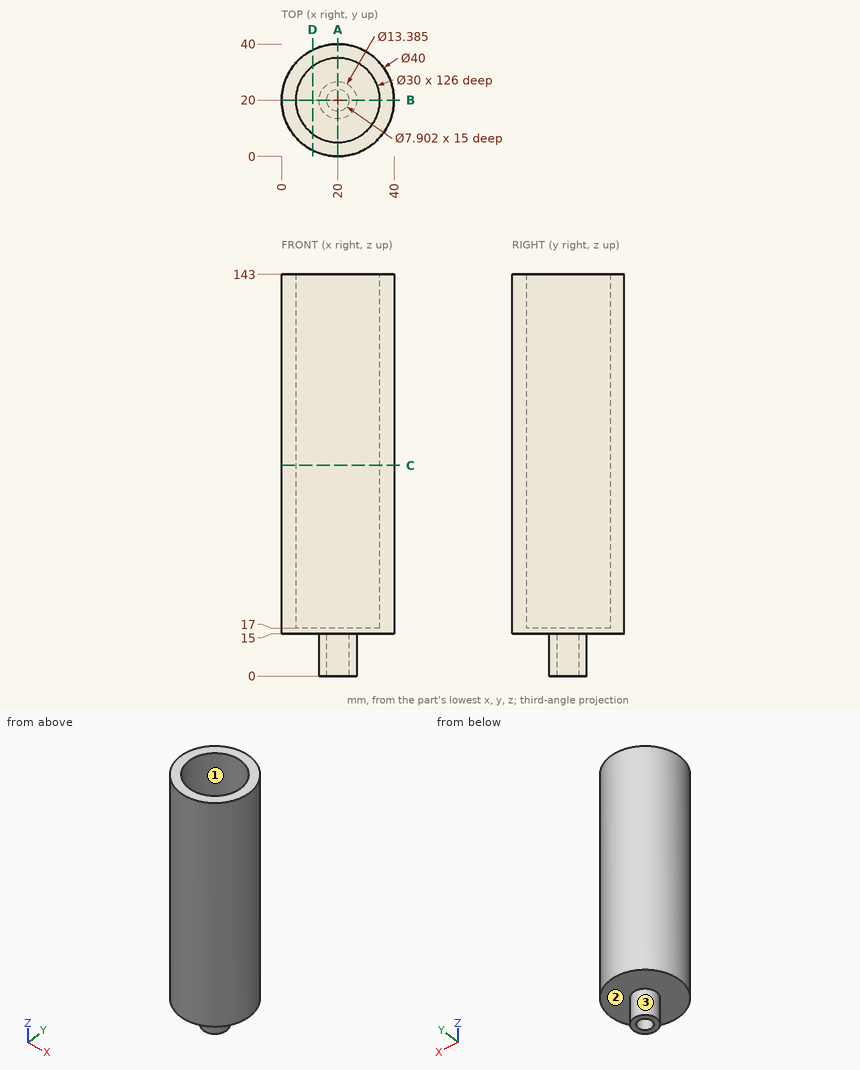
Here's the drawing with two shaded views (mm, measured from the low corner). I have some questions. Give positions to 0.01 mm unless a question says otherwise; leave off trailing zeros. Order: outer loops, then holes, each group sorted by start corner. A loop starts at its lowest first (then second) coordinate and runs counter-clockwise, first axis right, second up. Notation, with made-up numbers: (46, 66.25) - (105, 66.25) arc R35 cw to (105, 104.25) - close; hole circle Ø6 at (-20, 13.5). An arc over 180 degrees is marked (long way). Use a Markdown table: item, result. Add a question column.
Q1. If we section it at C-C on z = 75: Write out the boundary of the cut face in (x, y), plus the area to 3 significant figures.
Q2. If we section it at A-A on x = 20: Write out the boundary of the cut face in (y, z).
Q3. I'm going to push flat-ended pins straight in: pin 1 (4 mm diameter, centred on x = 27.5, z = 102.5, fed in from -Y); pin 2 (6.5 mm diameter, centred on x = 19, y = 18.5, fed in from -Z); pin 3 (9 mm diameter, centred on x = 17.5, y = 16, fed in from +Z); pin 4 (12 mm diameter, centred on x = 35, y = 21, fed in from -Z). Where does each tip first touch, or does it pass through?
Q4. Please list where these lines run through material, in increasing order: line 1 along X through (y, z) = (20, 10); line 2 along Y through (x, z) = (20, 77).
Q5. If we section it at D-D on x = 11: Write out the boundary of the cut face in (y, z), plus the area to 3 significant figures.
Q6. If we mould it in two halves opening along X, with no side actions, what happens to the marked faces 1, 2 and 3? For each: released by +X, released by -X, zero draft, split by the parting line, or undercut.
Answers follow:
| question | item | result |
|---|---|---|
| 1 | outline | circle Ø40 at (20, 20); hole circle Ø30 at (20, 20) |
| 1 | area | 550 mm^2 |
| 2 | outline | (0, 15) - (13.31, 15) - (13.31, 0) - (16.05, 0) - (16.05, 15) - (23.95, 15) - (23.95, 0) - (26.69, 0) - (26.69, 15) - (40, 15) - (40, 143) - (35, 143) - (35, 17) - (5, 17) - (5, 143) - (0, 143) - close |
| 3 | pin 1 | stops at y = 0.77 |
| 3 | pin 2 | stops at z = 0 |
| 3 | pin 3 | stops at z = 17 |
| 3 | pin 4 | stops at z = 15 |
| 4 | line 1 | x = 13.31 to 16.05, 23.95 to 26.69 |
| 4 | line 2 | y = 0 to 5, 35 to 40 |
| 5 | outline | (2.14, 15) - (37.86, 15) - (37.86, 143) - (32, 143) - (32, 17) - (8, 17) - (8, 143) - (2.14, 143) - close |
| 5 | area | 1,550 mm^2 |
| 6 | face 1 | undercut |
| 6 | face 2 | zero draft |
| 6 | face 3 | split by the parting line |
